Build history of the part. All positions in model axes, mm. Give positions to 0.01 mm unless a question says otherwise; leave off trailing zeros. Write each loop counter-clockwise with the first axis right and the second up, starting at its lowest first coordinate (ties: lowest second). Pieces come first, ordered by that corner, then holes. Notation, with made-up numbers: (9, 7.5) -> (34, 7.5) arc R13 ccw to (34, 26.5) -> close; hole circle Ø3 at (-13.5, -21). An arc over 180 degrees is marked (long way). Put each result on its own line as item: value. Start each with the question number.
Item 1: Slice it at A-A, the plane x = 0. List the corners of the cut face in (y, z) (3 decimals), plus the area to 3 significant figures.
Item 2: Slice it at B-B, the plane y = 5.25. Give the number of separate pieces and of enclosed holes in the cut face, plus the area to 3 significant figures.
Item 3: Flat gauge pins, fed straight in: pin 1 Ø14 at (x, z) = (30, -30) entering from +Y; pin 2 Ø1.5 at (x, y) = (-5.5, 5.5) entering from +Z. Where does each tip first touch, or does it go through?
Item 4: Drill centre lines: line 1 along X through (y, z) = (2.25, 0) (3 decimals); line 2 along Z through (x, y) = (-39, 2); line 3 along X through (y, z) = (1.75, -23.5). Where is each one in solid material? Low to high.
```python
from build123d import *

# Parameters (mm, degrees)
SKETCH1_R               = 76.2
BOSS_EXTRUDE1_DEPTH     = 6.35
CUT_EXTRUDE3_DEPTH      = 108.95
CUT_EXTRUDE3_DEPTH_BACK = 108.95
SKETCH3_R               = 10.025
SKETCH3_R_2             = 3.675
SKETCH3_R_3             = 11.6125


with BuildPart() as part:
    # Sketch1 → Boss-Extrude1 (new body)
    with BuildSketch(Plane(origin=(0, 0, 0), x_dir=(1, 0, 0), z_dir=(0, 1, 0))):
        with Locations(Location((0, 0, 0), (0, 0, 270))):
            Circle(SKETCH1_R)
    extrude(amount=BOSS_EXTRUDE1_DEPTH)

    # Sketch3 → Cut-Extrude3 (cut, two sides: drawn at the far end of the back side and taken through both)
    with BuildSketch(Plane(origin=(0, 0, 0), x_dir=(1, 0, 0), z_dir=(0, 1, 0)).offset(-CUT_EXTRUDE3_DEPTH_BACK)):
        with Locations(Location((-30, 30, 0), (0, 0, 270))):
            Circle(SKETCH3_R)
        with Locations(Location((30, -30, 0), (0, 0, 270))):
            Circle(SKETCH3_R)
        with Locations(Location((0, 30, 0), (0, 0, 270))):
            Circle(SKETCH3_R_2)
        with Locations(Location((30, 0, 0), (0, 0, 270))):
            Circle(SKETCH3_R_2)
        with Locations(Location((0, -30, 0), (0, 0, 270))):
            Circle(SKETCH3_R_2)
        with Locations(Location((-30, 0, 0), (0, 0, 270))):
            Circle(SKETCH3_R_2)
        with Locations(Location((30, 30, 0), (0, 0, 270))):
            Circle(SKETCH3_R_3)
        with Locations(Location((-30, -30, 0), (0, 0, 270))):
            Circle(SKETCH3_R_3)
    extrude(amount=CUT_EXTRUDE3_DEPTH + CUT_EXTRUDE3_DEPTH_BACK, mode=Mode.SUBTRACT)


solid = part.part
```
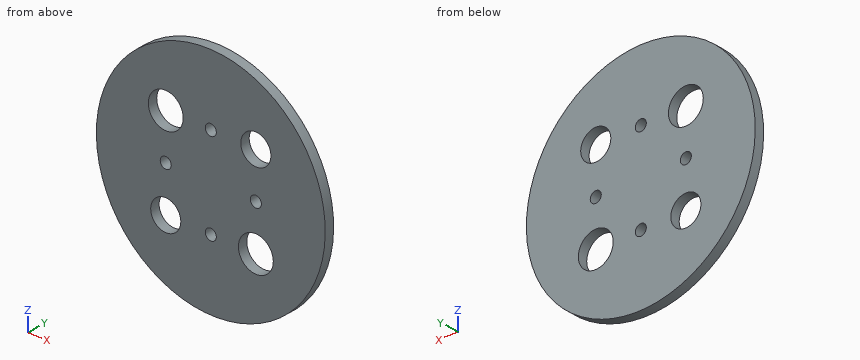
Values follow:
1. outline: (0, -76.2) -> (6.35, -76.2) -> (6.35, -33.675) -> (0, -33.675) -> close; (0, -26.325) -> (6.35, -26.325) -> (6.35, 26.325) -> (0, 26.325) -> close; (0, 33.675) -> (6.35, 33.675) -> (6.35, 76.2) -> (0, 76.2) -> close
1. area: 874 mm2
2. separate pieces: 1
2. enclosed holes: 8
2. area: 16,600 mm2
3. pin 1: through
3. pin 2: z = 76.05
4. line 1: -76.2 to -33.675, -26.325 to 26.325, 33.675 to 76.2
4. line 2: -65.46 to -34.42, -25.58 to 22.66, 37.34 to 65.46
4. line 3: -72.49 to -37.63, -22.37 to 20.38, 39.62 to 72.49
